Work out the finished part from the listing and answer in its coordinate system (mm). Face numbers are marked on the shaded views. A direction names the side the tool comes from. Coordinates: 2 decimals unless noted, no trailing zeros. Order: outer loops, then holes, each group sorted by start corner. A loop starts at its lowest first (then second) coordinate and runs counter-clockwise, first axis right, second up. Notation, with made-up numbers: (66.5, 75) - (115.5, 75) arc R9 ccw to (115.5, 85) - close; hole circle Ø3 at (75.25, -22). An arc over 180 degrees is marked (long way). Use CSV: the item, a comma, the result in double quotes. Start each with the question number.
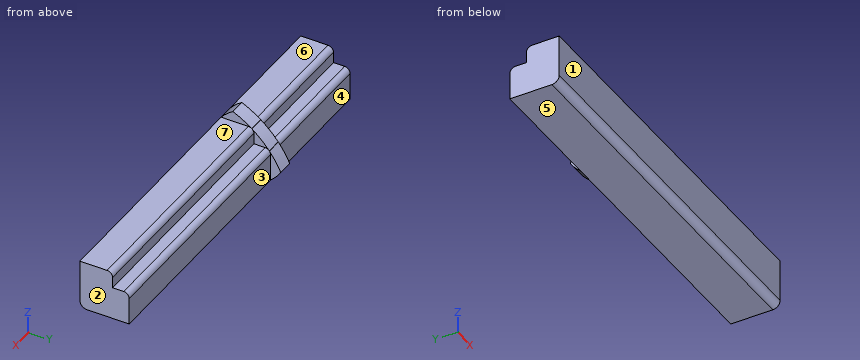
Autodesk Fusion 360 part; units mm, degrees
sketch "Sketch1" plane through (0, 0, 0) normal (0, 0, 1) x (1, 0, 0)
  line L0 (0, 0) -> (52, 0)
  line L1 (52, 0) -> (52, 6.7)
  line L2 (52, 6.7) -> (0, 6.7)
  line L3 (0, 6.7) -> (0, 0)
  dimension "d1" = 52
  dimension "d2" = 6.7
extrude "Extrude1" add sketch "Sketch1" along normal blind 6.7
sketch "Sketch2" plane through (0, 0, 6.7) normal (0, 0, 1) x (-1, 0, 0)
  line L0 (0, -6.7) -> (0, 0)
  line L1 (0, 0) -> (-52, 0)
  line L2 (-52, 0) -> (-52, -6.7)
  line L3 (-52, -6.7) -> (0, -6.7)
  line L4 (0, 0) -> (-52, 0)
  line L5 (-52, 0) -> (-52, -4.45)
  line L6 (-52, -4.45) -> (0, -4.45)
  line L7 (0, -4.45) -> (0, 0)
  dimension "d5" = 4.45
extrude "Extrude2" cut sketch "Sketch2" against normal blind 2.25 contours L0 L2 L3 L6
fillet "Fillet2" radius 0.75 2 edges at (26, 6.7, 4.45) (26, 4.45, 6.7)
fillet "Fillet3" radius 1 1 edges at (26, 0, 0)
ref_plane "WorkPlane2" through (18.75, 0, 0) normal (1, 0, 0) x (0, 1, 0)
sketch "Sketch8" plane through (18.75, 0, 0) normal (1, 0, 0) x (0, 1, 0)
  line L0 (4.45, 4.45) -> (6.7, 2.2) construction
  line L1 (4.45, 4.45) -> (2.1892, 6.7108) construction
  line L2 (0, 6.7) -> (1.6, 6.7) construction
  line L3 (6.7, 0) -> (6.7, 1.6) construction
  line L4 (6.7, 1.6) -> (8.1, 1.6) construction
  line L5 (1.6, 6.7) -> (1.6, 8.1) construction
  line L6 (4.45, 4.45) -> (7, 7) construction
  line L7 (5.575, 3.325) -> (8.1813, 5.9313) construction
  line L8 (3.3196, 5.5804) -> (5.5098, 7.7707) construction
  arc A0 (6.7, 0) -> (8.1, 1.6) centre (2.6, 5) ccw
  arc A1 (1.6, 8.1) -> (0, 6.7) centre (5, 2.6) ccw
  line L9 (0, 6.7) -> (6.7, 0)
  arc A2 (8.1, 1.6) -> (1.6, 8.1) centre (-4.0249, -4.0249) ccw
  dimension "d18" = 1.6
  dimension "d19" = 1.6
  dimension "d20" = 1.4
  dimension "d21" = 1.4
extrude "Extrude3" add sketch "Sketch8" against normal blind 2.1
1) The part is cut by section A-A on y = 2.25. Determine the outline of the cut face in (x, z), plus the area to 3 significant figures.
2) The part is cut by section B-B on x = 12.5. Determine the outline of the cut face in (y, z), plus the area to 3 significant figures.
3) The part is cut by section D-D on z = 7.5. Determine the outline of the cut face in (x, y), plus the area to 3 significant figures.
4) The part is cut by section C-C on z = 5. Determine the outline of the cut face in (x, y).
5) For the marked faces 4, 5, 6 and 7, determine the directions among +Z, -Z, +X, -X, +Y, -Y from which every point of the face is accessible in a straight line to the end or side of a thin tool.
6) For a pull along Y with two mould halves and no side action, classify the marked faces 1, 2 and 3 as +Y half, -Y half, draft (parallel to the pull), parting line (faces both ways), or undercut.
7) Flat-ended cylindrical pins translate along their axes: P1, Ø0.7, axis at y = 5, z = 5, coming from the -X side; P2, Ø3, axis at x = 37, y = 2, coming from the +Z side; P3, Ø1.2, axis at x = 33, z = 5.5, coming from the +Y side. Find the tip coordinate at first contact, or state that the pin passes through.
8) Straight lines are drawn through the part: line 1 (Y direction, x = 46.5, z = 1.75); line 2 (X direction, y = 5, z = 5.75). For each, find the intervals that lie inside material, in ascending order. Write a range as [from, to].
Answer key:
1,outline,"(0, 0) - (52, 0) - (52, 6.7) - (18.75, 6.7) - (18.75, 7.78) - (16.65, 7.78) - (16.65, 6.7) - (0, 6.7) - close"
1,area,"351 mm^2"
2,outline,"(0, 1) arc R1 ccw to (1, 0) - (6.7, 0) - (6.7, 3.7) arc R0.75 ccw to (5.95, 4.45) - (4.45, 4.45) - (4.45, 5.95) arc R0.75 ccw to (3.7, 6.7) - (0, 6.7) - close"
2,area,"39.4 mm^2"
3,outline,"(16.65, 0.78) - (18.75, 0.78) - (18.75, 2.74) - (16.65, 2.74) - close"
3,area,"4.12 mm^2"
4,outline,"(0, 0) - (52, 0) - (52, 4.45) - (18.75, 4.45) - (18.75, 5.83) - (16.65, 5.83) - (16.65, 4.45) - (0, 4.45) - close"
5,face 4,"+Z, -Z, -X, +Y"
5,face 5,"-Z, +X, -X, +Y, -Y"
5,face 6,"+Z, -X, +Y, -Y"
5,face 7,"+Z, +X, +Y, -Y"
6,face 1,"-Y half"
6,face 2,"draft"
6,face 3,"+Y half"
7,P1,"x = 16.65"
7,P2,"z = 6.7"
7,P3,"y = 4.45"
8,line 1,"[0, 6.7]"
8,line 2,"[16.65, 18.75]"
